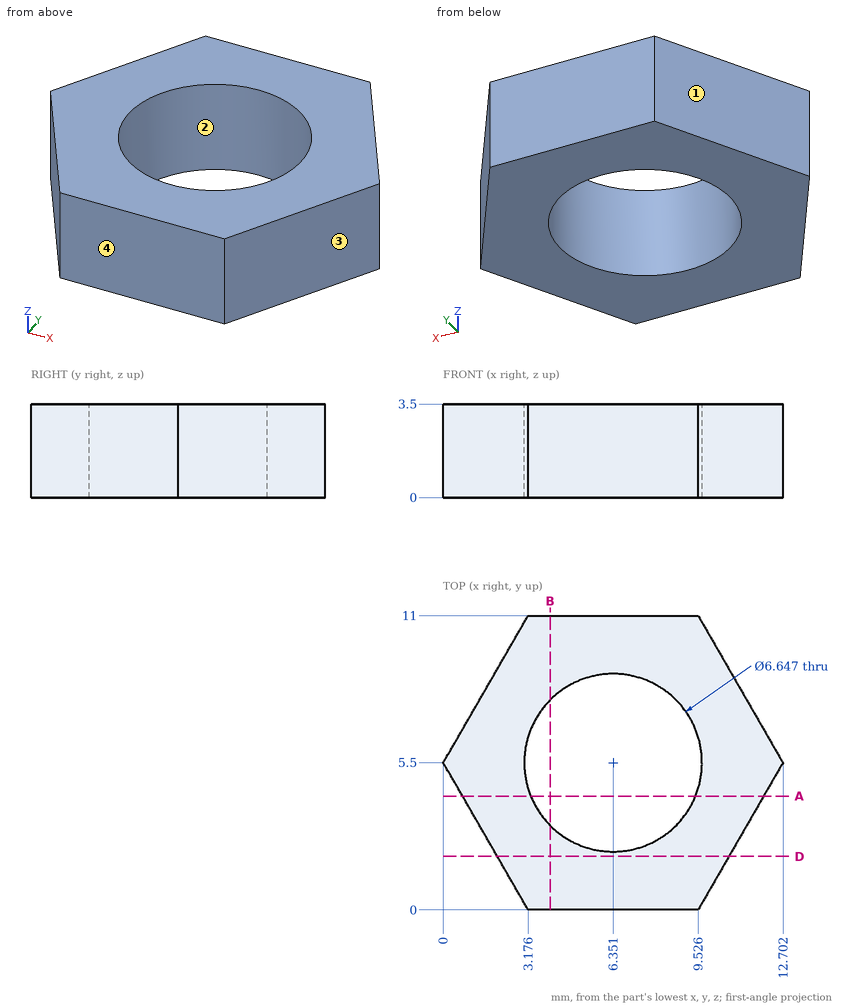
Could you check a few things on this drawing? It's one solid part, dimensions in mm from its lowest x, y, z. Give positions to 0.01 mm unless a question says otherwise; leave off trailing zeros. Order: outer loops, then holes, each group sorted by start corner. A loop starts at its lowest first (then second) coordinate and runs counter-clockwise, first axis right, second up. Notation, with made-up numbers: (60.5, 71.5) - (66.5, 71.5) arc R13 cw to (66.5, 91.5) - close; hole circle Ø9 at (-16.75, 21.25). An arc over 180 degrees is marked (long way). Return JSON: item names as keys, results as strings. Group by question number.
Q1. Thinking about a two-plate mould opening in X: for the marked faces 1, 2, 3 and 4, which applies, pulls with the +X half, pulls with the -X half, needs draft (parallel to the pull), parting line crosses it, or undercut?
Q2. Suppose I cut it at D-D, the plane y = 2. Please give me the cut outline in (x, z), and give its area (3 significant figures).
Q3. Please list where these lines run through material, in increasing order: line 1 along X through (y, z) = (6.5, 1.55) (1 decimal); line 2 along X through (y, z) = (5, 3.2) (1 decimal); line 3 along Y through (x, z) = (7, 0.5). Write a range as [from, to].
Q4. Suppose I cut it at B-B, the plane x = 4. Please give me the cut outline in (y, z).
Q5. Will this pin go through, and if not, where does the flat tip stop? pin 1 Ø1.5 at (x, y) = (8.5, 3.5) entering from +Z.
Q6. Suppose I cut it at A-A, the plane y = 4.25. Please give me the cut outline in (x, z).
Resolved:
{
 "1": {"face 1": "pulls with the -X half", "face 2": "undercut", "face 3": "pulls with the +X half", "face 4": "needs draft"},
 "2": {"outline": "(2.02, 0) - (10.68, 0) - (10.68, 3.5) - (2.02, 3.5) - close", "area": "30.3 mm2"},
 "3": {"line 1": "x = [0.6, 3.2], [9.5, 12.1]", "line 2": "x = [0.3, 3.1], [9.6, 12.4]", "line 3": "y = [0, 2.24], [8.76, 11]"},
 "4": {"outline": "(0, 0) - (3.15, 0) - (3.15, 3.5) - (0, 3.5) - close; (7.85, 0) - (11, 0) - (11, 3.5) - (7.85, 3.5) - close"},
 "5": {"pin 1": "stops at z = 3.5"},
 "6": {"outline": "(0.72, 0) - (3.27, 0) - (3.27, 3.5) - (0.72, 3.5) - close; (9.43, 0) - (11.98, 0) - (11.98, 3.5) - (9.43, 3.5) - close"}
}
